```python
from build123d import *

# Parameters (mm, degrees)
SKETCH1_W           = 273
SKETCH1_H           = 122
BOSS_EXTRUDE1_DEPTH = 5
SKETCH2_W           = 19
SKETCH2_H           = 96
BOSS_EXTRUDE2_DEPTH = 5
SKETCH3_W           = 6
SKETCH3_H           = 20
CUT_EXTRUDE1_DEPTH  = 6
SKETCH6_W           = 117.5
SKETCH6_H           = 2
CUT_EXTRUDE3_DEPTH  = 6
CUT_EXTRUDE4_DEPTH  = 10
SKETCH8_W           = 10
SKETCH8_H           = 10
CUT_EXTRUDE5_DEPTH  = 10


with BuildPart() as part:
    # Sketch1 → Boss-Extrude1 (new body)
    with BuildSketch(Plane.XY):
        Rectangle(SKETCH1_W, SKETCH1_H)
    extrude(amount=BOSS_EXTRUDE1_DEPTH)

    # Sketch2 → Boss-Extrude2 (add)
    with BuildSketch(Plane.XY.offset(5)):
        with Locations((-127, 109)):
            Rectangle(SKETCH2_W, SKETCH2_H)
    extrude(amount=-BOSS_EXTRUDE2_DEPTH)

    # Sketch3 → Cut-Extrude1 (cut)
    with BuildSketch(Plane.XY.offset(5)):
        with Locations((-114.5, 29)):
            Rectangle(SKETCH3_W, SKETCH3_H)
        with Locations((-114.5, -1)):
            Rectangle(SKETCH3_W, SKETCH3_H)
        with Locations((-114.5, -31)):
            Rectangle(SKETCH3_W, SKETCH3_H)
        with Locations((133.5, 29)):
            Rectangle(SKETCH3_W, SKETCH3_H)
        with Locations((133.5, -1)):
            Rectangle(SKETCH3_W, SKETCH3_H)
        with Locations((133.5, -31)):
            Rectangle(SKETCH3_W, SKETCH3_H)
    extrude(amount=-CUT_EXTRUDE1_DEPTH, mode=Mode.SUBTRACT)

    # Sketch6 → Cut-Extrude3 (cut)
    with BuildSketch(Plane.XY.offset(5)):
        with Locations((-58.75, 60)):
            Rectangle(SKETCH6_W, SKETCH6_H)
    extrude(amount=-CUT_EXTRUDE3_DEPTH, mode=Mode.SUBTRACT)

    # Sketch7 → Cut-Extrude4 (cut)
    with BuildSketch(Plane.XY.offset(5)):
        with BuildLine():
            ThreePointArc((-80.670694004, -51), (-84.938460957, -49.232233047), (-83.170694004, -53.5))
            Line((-83.170694004, -53.5), (-83.170694004, -51))
            Line((-83.170694004, -51), (-80.670694004, -51))
        make_face()
        with BuildLine():
            Line((-83.170694004, -51), (-83.170694004, -53.5))
            ThreePointArc((-83.170694004, -53.5), (-81.402927051, -52.767766953), (-80.670694004, -51))
            Line((-80.670694004, -51), (-83.170694004, -51))
        make_face()
        with BuildLine():
            ThreePointArc((-55.670694004, -51), (-54.938460957, -52.767766953), (-53.170694004, -53.5))
            Line((-53.170694004, -53.5), (-53.170694004, -51))
            Line((-53.170694004, -51), (-55.670694004, -51))
        make_face()
        with BuildLine():
            Line((-53.170694004, -51), (-53.170694004, -53.5))
            ThreePointArc((-53.170694004, -53.5), (-51.402927051, -52.767766953), (-50.670694004, -51))
            ThreePointArc((-50.670694004, -51), (-53.170694004, -48.5), (-55.670694004, -51))
            Line((-55.670694004, -51), (-53.170694004, -51))
        make_face()
    extrude(amount=-CUT_EXTRUDE4_DEPTH, mode=Mode.SUBTRACT)

    # Sketch8 → Cut-Extrude5 (cut)
    with BuildSketch(Plane.XY.offset(5)):
        with Locations((-11.5, -56)):
            Rectangle(SKETCH8_W, SKETCH8_H)
    extrude(amount=-CUT_EXTRUDE5_DEPTH, mode=Mode.SUBTRACT)


solid = part.part
```
Check sheet for the modelled part. Datum: model origin and axes. Units: mm. Round coordinates to 2 decimals unless told otherwise and drop trailing zeros. Loops run counter-clockwise (first coordinate to the right, second up) from the corner with the lowest first, then second, coordinate; pieces in that order, holes last. Notation, with made-up numbers: (24.5, 69.5) - (72.5, 69.5) arc R30 cw to (72.5, 100.5) - close; hole circle Ø10 at (22.25, -35). An arc over 180 degrees is marked (long way). Write item = value, one per line. Start each with the question number.
Q1. Thickness scan on L1, parallel to Y at x = -113, z = 2.35; L2, parallel to X at y = -23.5, z = 1.45; L3, parallel to X at y = 121.5, z = 0.8. Record the ranges inside material, lowest first.
Q2. Section check B-B (y = 107). Record the boundary of the cut face in (x, z), plus the area to 3 significant figures.
Q3. Depth check by flat-ended pin: P1, Ø10, axis at x = -23, y = 66, coming from the -Z side; P2, Ø2.5, axis at x = -63, z = 1.5, coming from the +Y side; P3, Ø1, axis at y = 80.5, z = 2, coming from the +X side. Enter the tip coordinate at first touch or a pass-through.
Q4. Section check C-C (z = 2.7). Count the separate pieces of the cut face and the enclosed holes in it, plus the area to 3 significant figures.
Q5. Section check A-A (y = 23). Record the boundary of the cut face in (x, z), plus the area to 4 significant figures.
Derived:
q1.L1 = -61 to -41, -21 to -11, 9 to 19, 39 to 59
q1.L2 = -136.5 to -117.5, -111.5 to 130.5
q1.L3 = -136.5 to -117.5
q2.outline = (-136.5, 0) - (-117.5, 0) - (-117.5, 5) - (-136.5, 5) - close
q2.area = 95.0 mm^2
q3.P1 = through
q3.P2 = 59
q3.P3 = -117.5
q4.separate_pieces = 1
q4.enclosed_holes = 5
q4.area = 34,000 mm^2
q5.outline = (-136.5, 0) - (-117.5, 0) - (-117.5, 5) - (-136.5, 5) - close; (-111.5, 0) - (130.5, 0) - (130.5, 5) - (-111.5, 5) - close
q5.area = 1,305 mm^2
